Geometry check sheet. Reference: the model listing, model coordinates, mm. Round coordinates to 2 decimals unless told otherwise and drop trailing zeros. Order: outer loops, then holes, each group sorted by start corner. A loop starts at its lowest first (then second) coordinate and runs counter-clockwise, first axis right, second up. Notation, with made-up numbers: (-40, 1) - (-20, 1) arc R25 ccw to (-20, 34) - close; hole circle Ø5 at (58, 68). An arc over 180 degrees is marked (long way). One line per question, with ' | ' between items. Start each with the question number.
Q1. Sectioned sample at D-D, the plane y = -141.5. Enter the section's corners in (x, z), then the cut area to 3 significant figures.
Q2. Gauge pin test, flat ends, axial feed: P1, Ø1.5, axis at y = -137.5, z = 1.5, coming from the -X side; P2, Ø4, axis at x = 63.5, y = -20.701, coming from the -Z side. Record the tip position at first contact, or that the pin passes through.
Q3. Sectioned sample at C-C, the plane z = 2.35. Give the number of separate pieces and of enclosed holes in the cut face, then the cut area to 3 significant figures.
Q4. Sectioned sample at B-B, the plane x = 165.1. Enter the section's corners in (y, z).
Q5. Material ranges on line 1 along Y through (x, z) = (114.3, 1.2); line 2 along X through (y, z) = (-20.5, 2.3); line 3 along Y through (x, z) = (117, 1.2), recorded low to high.
Q6. Sectioned sample at A-A, the plane x = 114.3. Enter the section's corners in (y, z).
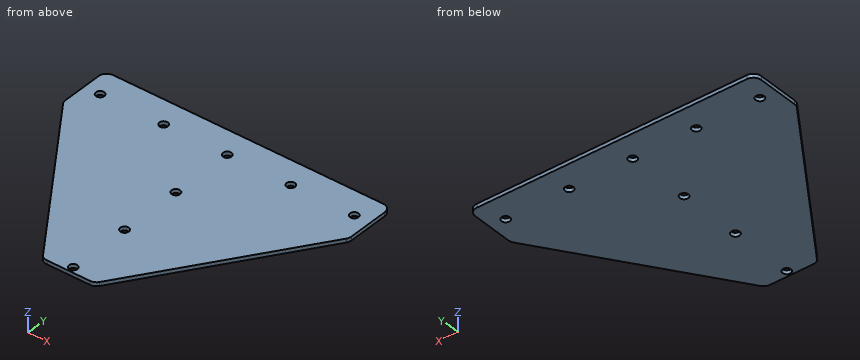
Autodesk Inventor part; units mm, degrees
ref_plane "YZ Plane" through (0, 0, 0) normal (1, 0, 0) x (0, 1, 0)
ref_plane "XZ Plane" through (0, 0, 0) normal (0, 1, 0) x (-1, 0, 0)
ref_plane "XY Plane" through (0, 0, 0) normal (0, 0, 1) x (1, 0, 0)
sketch "Sketch1" plane through (0, 0, 0) normal (0, 0, 1) x (1, 0, 0)
  line L0 (0, 0) -> (228.6, 0)
  line L1 (0, 0) -> (0, -41.402)
  line L2 (228.6, 0) -> (228.6, -41.402)
  line L3 (93.599, -177.8) -> (135.001, -177.8)
  line L4 (0, -41.402) -> (93.599, -177.8)
  line L5 (228.6, -41.402) -> (135.001, -177.8)
  circle A0 centre (215.9, -20.701) radius 3.3655
  circle A1 centre (165.1, -20.701) radius 3.3655
  circle A2 centre (114.3, -20.701) radius 3.3655
  circle A3 centre (63.5, -20.701) radius 3.3655
  circle A4 centre (12.7, -20.701) radius 3.3655
  line L6 (114.3, 0) -> (114.3, -20.701)
  circle A5 centre (114.3, -71.501) radius 3.3655
  circle A6 centre (114.3, -122.301) radius 3.3655
  circle A7 centre (114.3, -173.101) radius 3.3655
  dimension "d0" = 228.6
  dimension "d6" = 41.402
  dimension "d7" = 41.402
  dimension "d8" = 41.402
  dimension "d9" = 177.8
  dimension "d11" = 93.599
  dimension "d13" = 6.731
  dimension "d14" = 12.7
  dimension "d15" = 20.701
  dimension "d18" = 50.8
  dimension "d25" = 50.8
extrude "Plate1" add sketch "Sketch1" along normal blind 3.048
fillet "Corner Round1" radius 6.35 6 edges at (0, 0, 1.524) (0, -41.402, 1.524) (228.6, 0, 1.524) (228.6, -41.402, 1.524) (135.001, -177.8, 1.524) (93.599, -177.8, 1.524)
equation "\"d15\" = 0.5 * d6"
equation "\"BendRadius\" = Thickness"
equation "\"BendReliefWidth\" = Thickness"
equation "\"BendReliefDepth\" = 0.5 * Thickness"
equation "\"CornerReliefSize\" = 4 * Thickness"
equation "\"MinimumRemnant\" = 2 * Thickness"
equation "\"TransitionRadius\" = BendRadius"
equation "\"JacobiRadiusSize\" = BendRadius"
equation "\"GapSize\" = Thickness"
equation "\"d30\" = BendRadius"
properties part number "super4"
Determined:
1) outline: (68.69, 0) - (159.91, 0) - (159.91, 3.05) - (68.69, 3.05) - close | area: 278 mm2
2) P1: stops at x = 65.43 | P2: passes through
3) separate pieces: 1 | enclosed holes: 8 | area: 27,600 mm2
4) outline: (-133.94, 0) - (-24.07, 0) - (-24.07, 3.05) - (-133.94, 3.05) - close; (-17.34, 0) - (0, 0) - (0, 3.05) - (-17.34, 3.05) - close
5) line 1: y = -177.8 to -176.47, -169.74 to -125.67, -118.94 to -74.87, -68.14 to -24.07, -17.34 to 0 | line 2: x = 0 to 9.34, 16.06 to 60.14, 66.86 to 110.94, 117.66 to 161.74, 168.46 to 212.54, 219.26 to 228.6 | line 3: y = -177.8 to -175.11, -171.09 to -124.31, -120.29 to -73.51, -69.49 to -22.71, -18.69 to 0
6) outline: (-177.8, 0) - (-176.47, 0) - (-176.47, 3.05) - (-177.8, 3.05) - close; (-169.74, 0) - (-125.67, 0) - (-125.67, 3.05) - (-169.74, 3.05) - close; (-118.94, 0) - (-74.87, 0) - (-74.87, 3.05) - (-118.94, 3.05) - close; (-68.14, 0) - (-24.07, 0) - (-24.07, 3.05) - (-68.14, 3.05) - close; (-17.34, 0) - (0, 0) - (0, 3.05) - (-17.34, 3.05) - close
